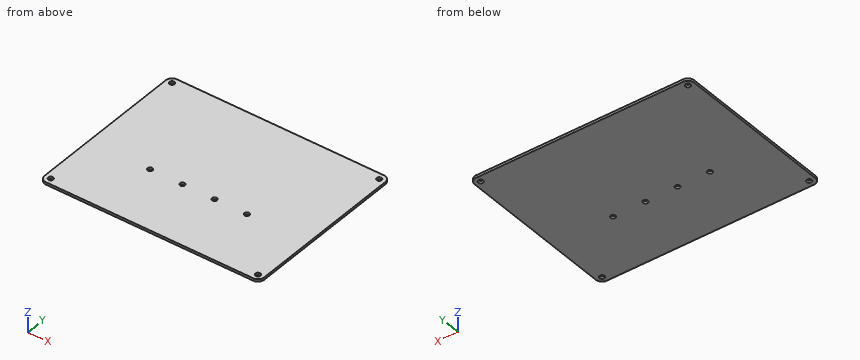
Autodesk Inventor part; units mm, degrees
ref_plane "YZ Plane" through (0, 0, 0) normal (1, 0, 0) x (0, 1, 0)
ref_plane "XZ Plane" through (0, 0, 0) normal (0, 1, 0) x (-1, 0, 0)
ref_plane "XY Plane" through (0, 0, 0) normal (0, 0, 1) x (1, 0, 0)
sketch "Sketch1" plane through (0, 0, 0) normal (0, 0, 1) x (1, 0, 0)
  line L0 (71.5, -55.5) -> (-71.5, -55.5)
  line L1 (-71.5, -55.5) -> (-71.5, 55.5)
  line L2 (-71.5, 55.5) -> (71.5, 55.5)
  line L3 (71.5, 55.5) -> (71.5, -55.5)
  line L4 (71.5, -55.5) -> (-71.5, 55.5) construction
  line L5 (-71.5, -55.5) -> (71.5, 55.5) construction
  point P0 (0, 0)
  dimension "d0" = 143
  dimension "d1" = 111
extrude "Extrusion1" add sketch "Sketch1" along normal blind 1.6
fillet "Fillet1" radius 4 4 edges at (71.5, 55.5, 0.8) (-71.5, 55.5, 0.8) (-71.5, -55.5, 0.8) (71.5, -55.5, 0.8)
sketch "Sketch2" plane through (0, 0, 1.6) normal (0, 0, 1) x (1, 0, 0)
  arc A0 (67.5, -55.5) -> (71.5, -51.5) centre (67.5, -51.5) ccw
  line L0 (71.5, -51.5) -> (71.5, 51.5)
  arc A1 (71.5, 51.5) -> (67.5, 55.5) centre (67.5, 51.5) ccw
  line L1 (67.5, 55.5) -> (-67.5, 55.5)
  arc A2 (-67.5, 55.5) -> (-71.5, 51.5) centre (-67.5, 51.5) ccw
  line L2 (-71.5, 51.5) -> (-71.5, -51.5)
  arc A3 (-71.5, -51.5) -> (-67.5, -55.5) centre (-67.5, -51.5) ccw
  line L3 (-67.5, -55.5) -> (67.5, -55.5)
  line L4 (-31.5, -14) -> (31.5, -14) construction
  line L5 (-10.5, -14) -> (10.5, -14) construction
  point P0 (0, 0)
  point P1 (0, -14)
  dimension "d9" = 21
  dimension "d17" = 21
  dimension "d18" = 41.5
hole "Hole1" at (-31.5, -14, 1.6) at (31.5, -14, 1.6) at (-10.5, -14, 1.6) at (10.5, -14, 1.6) at (-67.5, 51.5, 1.6) at (67.5, 51.5, 1.6) at (67.5, -51.5, 1.6) at (-67.5, -51.5, 1.6) direction (0, 0, -1) diameter 3.2 end through all
sketch "Sketch3" plane through (0, 0, 1.6) normal (0, 0, 1) x (1, 0, 0)
  line L0 (-67.5, -55.5) -> (67.5, -55.5)
  line L1 (-63, -20.5) -> (63, -20.5) construction
  point P0 (0, 0)
  point P1 (-42, -20.5)
  point P2 (-21, -20.5)
  point P3 (0, -20.5)
  point P4 (21, -20.5)
  point P5 (42, -20.5)
  dimension "d21" = 21
  dimension "d26" = 35
sketch "Sketch4" plane through (0, 0, 1.6) normal (0, 0, 1) x (1, 0, 0)
  circle A0 centre (63, -20.5) radius 8
  circle A1 centre (42, -20.5) radius 8
  circle A2 centre (21, -20.5) radius 8
  circle A3 centre (0, -20.5) radius 8
  circle A4 centre (-21, -20.5) radius 8
  circle A5 centre (-42, -20.5) radius 8
  circle A6 centre (-63, -20.5) radius 8
  circle A7 centre (-67.5, -51.5) radius 1.6
  circle A8 centre (67.5, -51.5) radius 1.6
  circle A9 centre (67.5, 51.5) radius 1.6
  circle A10 centre (-67.5, 51.5) radius 1.6
  circle A11 centre (10.5, -14) radius 1.6
  circle A12 centre (-10.5, -14) radius 1.6
  circle A13 centre (31.5, -14) radius 1.6
  circle A14 centre (-31.5, -14) radius 1.6
  arc A15 (67.5, -55.5) -> (71.5, -51.5) centre (67.5, -51.5) ccw
  line L0 (71.5, -51.5) -> (71.5, 51.5)
  arc A16 (71.5, 51.5) -> (67.5, 55.5) centre (67.5, 51.5) ccw
  line L1 (67.5, 55.5) -> (-67.5, 55.5)
  arc A17 (-67.5, 55.5) -> (-71.5, 51.5) centre (-67.5, 51.5) ccw
  line L2 (-71.5, 51.5) -> (-71.5, -51.5)
  arc A18 (-71.5, -51.5) -> (-67.5, -55.5) centre (-67.5, -51.5) ccw
  line L3 (-67.5, -55.5) -> (67.5, -55.5)
  line L4 (-63, -7.5096) -> (-51.75, -14.0048)
  line L5 (-51.75, -14.0048) -> (-51.75, -26.9952)
  line L6 (-51.75, -26.9952) -> (-63, -33.4904)
  line L7 (-63, -33.4904) -> (-74.25, -26.9952)
  line L8 (-74.25, -26.9952) -> (-74.25, -14.0048)
  line L9 (-74.25, -14.0048) -> (-63, -7.5096)
  line L10 (63, -7.5096) -> (74.25, -14.0048)
  line L11 (74.25, -14.0048) -> (74.25, -26.9952)
  line L12 (74.25, -26.9952) -> (63, -33.4904)
  line L13 (63, -33.4904) -> (51.75, -26.9952)
  line L14 (51.75, -26.9952) -> (51.75, -14.0048)
  line L15 (51.75, -14.0048) -> (63, -7.5096)
  point P0 (0, 0)
  point P1 (71.5, -12.4171)
  point P2 (71.5, -28.5829)
  point P3 (-71.5, -28.5829)
  point P4 (-71.5, -12.4171)
  dimension "d34" = 22.5
  dimension "d35" = 22.5
sketch "Sketch5" plane through (0, 0, 1.6) normal (0, 0, 1) x (1, 0, 0)
  line L0 (-42, -6) -> (42, -6) construction
  line L1 (-67.5, -55.5) -> (67.5, -55.5)
  circle A0 centre (-42, -20.5) radius 8
  circle A1 centre (-21, -20.5) radius 8
  circle A2 centre (0, -20.5) radius 8
  circle A3 centre (21, -20.5) radius 8
  circle A4 centre (42, -20.5) radius 8
  point P0 (0, 0)
  point P1 (0, -6)
  point P2 (0, -55.5)
  point P3 (-21, -6)
  point P4 (0, -6)
  point P5 (21, -6)
  dimension "d39" = 49.5
sketch "Sketch6" plane through (0, 0, 1.6) normal (0, 0, 1) x (1, 0, 0)
  line L0 (-67.5, -55.5) -> (67.5, -55.5) construction
  line L1 (-71.5, 51.5) -> (-71.5, -11.2624) construction
  point P0 (0, 0)
  point P1 (-68.5, 13.5)
  point P2 (-63.5, 13.5)
  point P3 (-58.5, 13.5)
  point P4 (-53.5, 13.5)
  dimension "d49" = 5
  dimension "d54" = 69
  dimension "d55" = 3
sketch "Sketch7" plane through (0, 0, 1.6) normal (0, 0, 1) x (1, 0, 0)
  circle A0 centre (-68.5, 13.5) radius 1.7
  line L0 (-68.5, 18.1188) -> (-64.5, 15.8094)
  line L1 (-64.5, 15.8094) -> (-64.5, 11.1906)
  line L2 (-64.5, 11.1906) -> (-68.5, 8.8812)
  line L3 (-68.5, 8.8812) -> (-72.5, 11.1906)
  line L4 (-72.5, 11.1906) -> (-72.5, 15.8094)
  line L5 (-72.5, 15.8094) -> (-68.5, 18.1188)
  line L6 (-71.5, 51.5) -> (-71.5, -11.2624)
  point P0 (0, 0)
  point P1 (-71.5, 10.6132)
  point P2 (-71.5, 16.3868)
  dimension "d63" = 1
sketch "Sketch8" plane through (0, 0, 1.6) normal (0, 0, 1) x (1, 0, 0)
  line L0 (68.5, 21.1) -> (34.5, 21.1)
  line L1 (34.5, 21.1) -> (34.5, 40.1)
  line L2 (34.5, 40.1) -> (68.5, 40.1)
  line L3 (68.5, 40.1) -> (68.5, 21.1)
  line L4 (68.5, 21.1) -> (34.5, 40.1) construction
  line L5 (34.5, 21.1) -> (68.5, 40.1) construction
  line L6 (71.5, -11.2624) -> (71.5, 51.5)
  line L7 (-67.5, -55.5) -> (67.5, -55.5)
  point P0 (0, 0)
  point P1 (51.5, 30.6)
  dimension "d67" = 20
  dimension "d68" = 86.1
  dimension "d69" = 34
  dimension "d70" = 19
sketch "Sketch9" plane through (0, 0, 1.6) normal (0, 0, 1) x (1, 0, 0)
  line L0 (67.25, 14.25) -> (35.75, 14.25)
  line L1 (35.75, 14.25) -> (35.75, 43.95)
  line L2 (35.75, 43.95) -> (67.25, 43.95)
  line L3 (67.25, 43.95) -> (67.25, 14.25)
  line L4 (67.25, 14.25) -> (35.75, 43.95) construction
  line L5 (35.75, 14.25) -> (67.25, 43.95) construction
  line L6 (-67.5, -55.5) -> (67.5, -55.5)
  point P0 (0, 0)
  point P1 (51.5, 29.1)
  point P2 (51.5, 30.6)
  dimension "d74" = 31.5
  dimension "d75" = 29.7
  dimension "d76" = 69.75
sketch "Sketch10" plane through (0, 0, 1.6) normal (0, 0, 1) x (1, 0, 0)
  circle A0 centre (35.75, 14.25) radius 3
  circle A1 centre (67.25, 14.25) radius 3
  circle A2 centre (67.25, 43.95) radius 3
  circle A3 centre (35.75, 43.95) radius 3
  line L0 (34.5, 22.1) -> (34.5, 39.1)
  arc A4 (35.5, 40.1) -> (34.5, 39.1) centre (35.5, 39.1) ccw
  line L1 (35.5, 40.1) -> (67.5, 40.1)
  arc A5 (68.5, 39.1) -> (67.5, 40.1) centre (67.5, 39.1) ccw
  line L2 (68.5, 39.1) -> (68.5, 22.1)
  arc A6 (67.5, 21.1) -> (68.5, 22.1) centre (67.5, 22.1) ccw
  line L3 (67.5, 21.1) -> (35.5, 21.1)
  arc A7 (34.5, 22.1) -> (35.5, 21.1) centre (35.5, 22.1) ccw
  circle A8 centre (-53.5, 13.5) radius 1.7
  circle A9 centre (-58.5, 13.5) radius 1.7
  circle A10 centre (-63.5, 13.5) radius 1.7
  circle A11 centre (-68.5, 13.5) radius 1.7
  circle A12 centre (42, -6) radius 2.75
  circle A13 centre (21, -6) radius 2.75
  circle A14 centre (0, -6) radius 2.75
  circle A15 centre (-21, -6) radius 2.75
  circle A16 centre (-42, -6) radius 2.75
  circle A17 centre (63, -20.5) radius 8
  circle A18 centre (42, -20.5) radius 8
  circle A19 centre (21, -20.5) radius 8
  circle A20 centre (0, -20.5) radius 8
  circle A21 centre (-21, -20.5) radius 8
  circle A22 centre (-42, -20.5) radius 8
  circle A23 centre (-63, -20.5) radius 8
  circle A24 centre (-67.5, -51.5) radius 1.6
  circle A25 centre (67.5, -51.5) radius 1.6
  circle A26 centre (67.5, 51.5) radius 1.6
  circle A27 centre (-67.5, 51.5) radius 1.6
  circle A28 centre (10.5, -14) radius 1.6
  circle A29 centre (-10.5, -14) radius 1.6
  circle A30 centre (31.5, -14) radius 1.6
  circle A31 centre (-31.5, -14) radius 1.6
  arc A32 (-72.5, 11.6236) -> (-72.125, 10.9741) centre (-71.75, 11.6236) ccw
  line L4 (-72.125, 10.9741) -> (-71.875, 10.8298)
  arc A33 (-71.5, 10.1802) -> (-71.875, 10.8298) centre (-72.25, 10.1802) ccw
  line L5 (-71.5, 10.1802) -> (-71.5, -11.2624)
  arc A34 (-72.5, -12.9944) -> (-71.5, -11.2624) centre (-73.5, -11.2624) ccw
  line L6 (-72.5, -12.9944) -> (-73.25, -13.4275)
  arc A35 (-73.25, -13.4275) -> (-74.25, -15.1595) centre (-72.25, -15.1595) ccw
  line L7 (-74.25, -15.1595) -> (-74.25, -25.8405)
  arc A36 (-74.25, -25.8405) -> (-73.25, -27.5725) centre (-72.25, -25.8405) ccw
  line L8 (-73.25, -27.5725) -> (-72.5, -28.0056)
  arc A37 (-71.5, -29.7376) -> (-72.5, -28.0056) centre (-73.5, -29.7376) ccw
  line L9 (-71.5, -29.7376) -> (-71.5, -51.5)
  arc A38 (-71.5, -51.5) -> (-67.5, -55.5) centre (-67.5, -51.5) ccw
  line L10 (-67.5, -55.5) -> (67.5, -55.5)
  arc A39 (67.5, -55.5) -> (71.5, -51.5) centre (67.5, -51.5) ccw
  line L11 (71.5, -51.5) -> (71.5, -29.7376)
  arc A40 (72.5, -28.0056) -> (71.5, -29.7376) centre (73.5, -29.7376) ccw
  line L12 (72.5, -28.0056) -> (73.25, -27.5725)
  arc A41 (73.25, -27.5725) -> (74.25, -25.8405) centre (72.25, -25.8405) ccw
  line L13 (74.25, -25.8405) -> (74.25, -15.1595)
  arc A42 (74.25, -15.1595) -> (73.25, -13.4275) centre (72.25, -15.1595) ccw
  line L14 (73.25, -13.4275) -> (72.5, -12.9944)
  arc A43 (71.5, -11.2624) -> (72.5, -12.9944) centre (73.5, -11.2624) ccw
  line L15 (71.5, -11.2624) -> (71.5, 51.5)
  arc A44 (71.5, 51.5) -> (67.5, 55.5) centre (67.5, 51.5) ccw
  line L16 (67.5, 55.5) -> (-67.5, 55.5)
  arc A45 (-67.5, 55.5) -> (-71.5, 51.5) centre (-67.5, 51.5) ccw
  line L17 (-71.5, 51.5) -> (-71.5, 16.8198)
  arc A46 (-71.875, 16.1702) -> (-71.5, 16.8198) centre (-72.25, 16.8198) ccw
  line L18 (-71.875, 16.1702) -> (-72.125, 16.0259)
  arc A47 (-72.125, 16.0259) -> (-72.5, 15.3764) centre (-71.75, 15.3764) ccw
  line L19 (-72.5, 15.3764) -> (-72.5, 11.6236)
  line L20 (67.25, 21.4669) -> (73.5, 17.8584)
  line L21 (73.5, 17.8584) -> (73.5, 10.6416)
  line L22 (73.5, 10.6416) -> (67.25, 7.0331)
  line L23 (67.25, 7.0331) -> (61, 10.6416)
  line L24 (61, 10.6416) -> (61, 17.8584)
  line L25 (61, 17.8584) -> (67.25, 21.4669)
  line L26 (67.25, 51.1669) -> (73.5, 47.5584)
  line L27 (73.5, 47.5584) -> (73.5, 40.3416)
  line L28 (73.5, 40.3416) -> (67.25, 36.7331)
  line L29 (67.25, 36.7331) -> (61, 40.3416)
  line L30 (61, 40.3416) -> (61, 47.5584)
  line L31 (61, 47.5584) -> (67.25, 51.1669)
  line L32 (73.5, 40.3416) -> (73.5, 17.8584)
  point P0 (0, 0)
  point P1 (71.5, 48.7131)
  point P2 (71.5, 9.4869)
  dimension "d84" = 2
equation "\"d35\" = d34"
properties part number "bot_cover_template"
Input: part model. Units: mm. Frame: model coordinates. Give positions to 0.01 mm unless a question says otherwise; leave off trailing zeros. Order: outer loops, then holes, each group sorted by start corner. A loop starts at its lowest first (then second) coordinate and runs counter-clockwise, first axis right, second up. Notation, with made-up numbers: (-39, -13.75) - (13, -13.75) arc R25 ccw to (13, 5.25) - close; hole circle Ø2 at (57, 82.25). An arc over 180 degrees is marked (long way). Put each result on its own line as item: value.
Item 1: Contact query for flat-ended pins moving along their axis: pin 1 (5 mm diameter, centred on x = -67.5, y = 51.5, fed in from +Z); pin 2 (1.9 mm diameter, centred on x = -31.5, y = -14, fed in from -Z). Output: stop coordinate, or through.
Found:
pin 1: stops at z = 1.6
pin 2: passes through
Item 2: Section query A-A, the plane y = -14. Return loops of the section in (x, z), then the cut area to 3 significant figures.
Found:
outline: (-71.5, 0) - (-33.1, 0) - (-33.1, 1.6) - (-71.5, 1.6) - close; (-29.9, 0) - (-12.1, 0) - (-12.1, 1.6) - (-29.9, 1.6) - close; (-8.9, 0) - (8.9, 0) - (8.9, 1.6) - (-8.9, 1.6) - close; (12.1, 0) - (29.9, 0) - (29.9, 1.6) - (12.1, 1.6) - close; (33.1, 0) - (71.5, 0) - (71.5, 1.6) - (33.1, 1.6) - close
area: 208 mm^2
Item 3: Ray query, L1, parallel to X at y = -14, z = 1.2; L2, parallel to Y at x = 67.5, z = 1.1; L3, parallel to Y at x = -31.5, z = 0.6. Return the intervals inside material, ascending. Write a range as from..to.
Found:
L1: x = -71.5..-33.1, -29.9..-12.1, -8.9..8.9, 12.1..29.9, 33.1..71.5
L2: y = -55.5..-53.1, -49.9..49.9, 53.1..55.5
L3: y = -55.5..-15.6, -12.4..55.5
Item 4: Section query B-B, the plane x = 31.5. Return loops of the section in (y, z), then the cut area to 3 significant figures.
Found:
outline: (-55.5, 0) - (-15.6, 0) - (-15.6, 1.6) - (-55.5, 1.6) - close; (-12.4, 0) - (55.5, 0) - (55.5, 1.6) - (-12.4, 1.6) - close
area: 172 mm^2
